from build123d import *

# Parameters (mm, degrees)
F0_R     = 38.9255
F0_R_2   = 3.46075
F0_R_3   = 13.97
F1_DEPTH = 5.2324
F0_R_4   = 9.0805
F2_DEPTH = 14.224
F3_R     = 2.54
F5_SIZE  = 2.54


# Not quite as in the source:
# - a fillet or chamfer that OpenCascade refuses, or shapes differently, is made with other operations: its cross-section is extruded or revolved along the edge and cut away or added


with BuildPart() as f1:
    # F0 (on Top) → F1 (new body)
    with BuildSketch(Plane.XY):
        Circle(F0_R)
        with Locations((0, -27.01925)):
            Circle(F0_R_2, mode=Mode.SUBTRACT)
        with Locations((-27.01925, 0)):
            Circle(F0_R_2, mode=Mode.SUBTRACT)
        Circle(F0_R_3, mode=Mode.SUBTRACT)
        with Locations((27.01925, 0)):
            Circle(F0_R_2, mode=Mode.SUBTRACT)
        with Locations((0, 27.01925)):
            Circle(F0_R_2, mode=Mode.SUBTRACT)
    extrude(amount=F1_DEPTH)

    # F0 (on Top) → F2 (join)
    with BuildSketch(Plane.XY):
        Circle(F0_R_3)
        Circle(F0_R_4, mode=Mode.SUBTRACT)
    extrude(amount=F2_DEPTH)

    # F3
    f3_edges = [f1.edges().sort_by_distance(p)[0] for p in [
        (-38.9255, 0, 5.2324),
        (-13.97, 0, 14.224),
        (-13.97, 0, 5.2324),
    ]]
    fillet(f3_edges, radius=F3_R)

    # F4: fillet of radius 2.54 on 1 edges, made by hand

    # F4_s1 → F4_t2 (revolve, cut)
    with BuildSketch(Plane.XZ):
        with BuildLine():
            ThreePointArc((9.0805, 11.6911538243), (9.7583144561, 13.4185405789), (11.43, 14.224))
            Line((11.43, 14.224), (9.0805, 14.224))
            Line((9.0805, 14.224), (9.0805, 11.6911538243))
        make_face()
    revolve(axis=Axis((0, 0, 14.224), (0, 0, 1)), mode=Mode.SUBTRACT)

    # F5
    f5_edges = [f1.edges().sort_by_distance(p)[0] for p in [
        (-3.46075, 27.01925, 5.2324),
        (23.5585, 0, 5.2324),
        (-3.46075, -27.01925, 5.2324),
        (-30.48, 0, 5.2324),
    ]]
    chamfer(f5_edges, length=F5_SIZE)


solid = f1.part
Part model, mm, in its own coordinate system. A direction names the side the tool comes from. Coordinates: 2 decimals unless noted, no trailing zeros. Loops run counter-clockwise (first coordinate to the right, second up) from the corner with the lowest first, then second, coordinate; pieces in that order, holes last. Notation, with made-up numbers: (-11, 33) - (-4, 33) arc R12 ccw to (-4, 54) - close; hole circle Ø7 at (-15.75, 14.25). An arc over 180 degrees is marked (long way). Write each question's results on one line, items separated by ' | '. Start each with the question number.
Q1. Slice it at A-A on x = 0. Give the number of separate pieces and of enclosed holes in the cut face, and give its area (3 significant figures).
Q2. Which spindle directions (+Z, -Z, +X, -X, +Y, -Y) get a long thin tool onto all of the face, cutting with end or side? Do faces 1 (the cylindrical face through (-1.82, 13.85, 9.7)), 2 (the cylindrical face through (23.56, 0.15, 1.33)). Say none if no direction does.
Q3. Probe line 1 along Y through (x, z) = (0, 1.3); line 2 along Z through (x, y) = (-20, 23); line 3 along Y through (x, z) = (0, 9.25). List the from-to ranges inside material, lowest first.
Q4. Slice it at C-C on z = 9.5. Give the cut face in (x, y), and give its area (3 significant figures).
Q5. Two-plate mould, pull along X, no slides. Class faces 3 (the conical face through (-0.467, -23.466, 2.816)), 4 (the flat face through (16, -8, 5.232)), 5 (the cylindrical face through (35.957, -14.909, 1.327)): +X half, -X half, draft (parallel to the pull), parting line (faces both ways), or undercut.
Q6. Drop flat-ended pins along their axis: pin 1 Ø5 at (x, y) = (3, -19.5) entering from -Z; pin 2 Ø4 at (x, z) = (-10, 8) entering from +Y; pin 3 Ø9 at (x, y) = (27.02, 0) entering from +Z; pin 4 Ø3 at (x, y) = (18.5, 8) entering from +Z. Give the stop position or say it passes through.
Answer:
1) separate pieces: 4 | enclosed holes: 0 | area: 309 mm2
2) face 1: +Z | face 2: +Z, -Z
3) line 1: y = -38.93 to -30.48, -23.56 to -9.08, 9.08 to 23.56, 30.48 to 38.93 | line 2: z = 0 to 5.23 | line 3: y = -13.97 to -9.08, 9.08 to 13.97
4) outline: circle Ø27.94 at (0, 0); hole circle Ø18.16 at (0, 0) | area: 354 mm2
5) face 3: undercut | face 4: draft | face 5: parting line
6) pin 1: stops at z = 0 | pin 2: stops at y = 11.45 | pin 3: stops at z = 3.73 | pin 4: stops at z = 5.23
